The listing builds one solid part. Answer for the finished solid, in the listing's coordinates (mm). Face numbers are marked on the shaded views. Round coordinates to 2 decimals unless told otherwise and drop trailing zeros. Loops run counter-clockwise (first coordinate to the right, second up) from the corner with the lowest first, then second, coordinate; pieces in that order, holes last. Notation, with made-up numbers: M 64,74.5 L 85,74.5 A34 cw 85,108.5 Z; hole C 44,6 d1. An arc over 180 degrees is marked long. Put each result on its own line as item: value. Start each with the question number.
(1) A flat-ended cylindrical pin translates along its axis: P1, Ø5, axis at x = -5, y = -6, coming from the -Z side. Find the tip coordinate at first contact, or state that the pin passes through.
(2) Section A-A, the plane x = 20.5 is taken. Determine the outline of the cut face in (y, z), then the cut area to 3 significant figures.
(3) Section B-B, the plane z = 5.5 is taken. Determine the outline of the cut face in (x, y), then the cut area to 3 significant figures.
(4) Straight lines are drawn through the part: line 1 (Z direction, x = 25, y = -9); line 2 (Z direction, x = 27, y = 11); line 3 (Y direction, x = 6.5, z = 3.5). For each, find the intervals that lie inside material, in ascending order.
(5) Section C-C, the plane y = 14.5 is taken. Determine the outline of the cut face in (x, z), then the cut area to 3 significant figures.
(6) Determine the mould class of the marked faces 1, 2 and 3 for opening direction Y: released by +Y, released by -Y, zero draft, split by the parting line, or undercut.
```python
from build123d import *

# Parameters (mm, degrees)
CROQUIS1_W              = 69
CROQUIS1_H              = 37
SALIENTE_EXTRUIR1_DEPTH = 19.5
CORTAR_EXTRUIR3_DEPTH   = 70


with BuildPart() as part:
    # Croquis1 → Saliente-Extruir1 (new body)
    with BuildSketch(Plane.XY):
        Rectangle(CROQUIS1_W, CROQUIS1_H)
    extrude(amount=SALIENTE_EXTRUIR1_DEPTH)

    # Croquis2 → Cortar-Extruir3 (cut)
    with BuildSketch(Plane(origin=(34.5, 0, 0), x_dir=(0, 0, -1), z_dir=(1, 0, 0))):
        with BuildLine():
            Line((0, 18.5), (-6.665805067, 18.5))
            ThreePointArc((-6.665805067, 18.5), (-1.896690737, 15.030939451), (0, 9.446908932))
            Line((0, 9.446908932), (0, 18.5))
        make_face()
        with BuildLine():
            Line((0, -9.053091068), (0, 9.053090641))
            ThreePointArc((0, 9.053090641), (-0.150040841, 7.534931091), (-0.535059254, 6.058759862))
            ThreePointArc((-0.535059254, 6.058759862), (-1.05, 0.19825397), (-0.677845098, -5.673048612))
            ThreePointArc((-0.677845098, -5.673048612), (-0.18835007, -7.332873528), (0, -9.053091068))
        make_face()
        with BuildLine():
            ThreePointArc((0, -9.446909359), (-1.896690336, -15.030939334), (-6.665803784, -18.5))
            Line((-6.665803784, -18.5), (0, -18.5))
            Line((0, -18.5), (0, -9.446909359))
        make_face()
    extrude(amount=-CORTAR_EXTRUIR3_DEPTH, mode=Mode.SUBTRACT)


solid = part.part
```
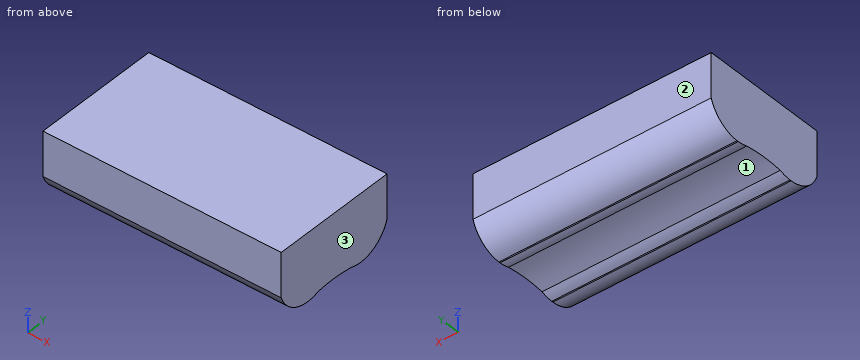
Recorded:
1. P1: stops at z = 0.03
2. outline: M -18.5,6.67 A9.75 ccw -9.45,0 L -9.05,0 A9.75 ccw -5.67,0.68 A39.01 cw 6.06,0.54 A9.75 ccw 9.05,0 L 9.45,0 A9.75 ccw 18.5,6.67 L 18.5,19.5 L -18.5,19.5 Z
2. area: 676 mm²
3. outline: M -34.5,-18.03 L 34.5,-18.03 L 34.5,18.03 L -34.5,18.03 Z
3. area: 2,490 mm²
4. line 1: z = 0 to 19.5
4. line 2: z = 0.16 to 19.5
4. line 3: y = -16.73 to 16.73
5. outline: M -34.5,1.53 L 34.5,1.53 L 34.5,19.5 L -34.5,19.5 Z
5. area: 1,240 mm²
6. face 1: undercut
6. face 2: released by +Y
6. face 3: zero draft
